from build123d import *

# Parameters (mm, degrees)
SKETCH1_W           = 250
SKETCH1_H           = 150
BOSS_EXTRUDE1_DEPTH = 4
SKETCH2_R           = 20
CUT_EXTRUDE1_DEPTH  = 4
SKETCH3_R           = 2
CUT_EXTRUDE2_DEPTH  = 4
SKETCH4_R           = 14.5
SKETCH4_R_2         = 1.8
CUT_EXTRUDE4_DEPTH  = 4


with BuildPart() as part:
    # Sketch1 → Boss-Extrude1 (new body)
    with BuildSketch(Plane.XY):
        with Locations((12.175324675, -10.633116883)):
            Rectangle(SKETCH1_W, SKETCH1_H)
    extrude(amount=BOSS_EXTRUDE1_DEPTH)

    # Sketch2 → Cut-Extrude1 (cut)
    with BuildSketch(Plane.XY.offset(4)):
        with Locations((12.175324675, -10.633116883)):
            Circle(SKETCH2_R)
    extrude(amount=-CUT_EXTRUDE1_DEPTH, mode=Mode.SUBTRACT)

    # Sketch3 → Cut-Extrude2 (cut)
    with BuildSketch(Plane.XY.offset(4)):
        with Locations((-3.824675325, 5.366883117)):
            Circle(SKETCH3_R)
        with Locations((28.175324675, 5.366883117)):
            Circle(SKETCH3_R)
        with Locations((28.175324675, -26.633116883)):
            Circle(SKETCH3_R)
        with Locations((-3.824675325, -26.633116883)):
            Circle(SKETCH3_R)
    extrude(amount=-CUT_EXTRUDE2_DEPTH, mode=Mode.SUBTRACT)

    # Sketch4 → Cut-Extrude4 (cut)
    with BuildSketch(Plane.XY.offset(4)):
        with Locations((-62.824675325, -55.633116883)):
            Circle(SKETCH4_R)
        with Locations((-74.824675325, -43.633116883)):
            Circle(SKETCH4_R_2)
        with Locations((-50.824675325, -67.633116883)):
            Circle(SKETCH4_R_2)
    extrude(amount=-CUT_EXTRUDE4_DEPTH, mode=Mode.SUBTRACT)


solid = part.part
Can you work these out from the model? Positions are in its coordinate system, mm. Coordinates: 2 decimals unless noted, no trailing zeros. Order: outer loops, then holes, each group sorted by start corner. A loop starts at its lowest first (then second) coordinate and runs counter-clockwise, first axis right, second up. Notation, with made-up numbers: (76, 29) - (131, 29) arc R20 cw to (131, 57) - close; hole circle Ø6 at (33, 83.25). An arc over 180 degrees is marked (long way). Answer as a JSON object with one key per item and string values. Group by question number.
Q1. Imagine slicing it at B-B (z = 2.25). Give the number of separate pieces and of enclosed holes in the cut face, and give its area (3 significant figures).
Q2. We'd pull the mould along X, two halves only. Please class faces 1 (the face through (30.65, -18.29, 2.03)), 2 (the face through (38, -10, 4)): +X half, -X half, draft (parallel to the pull), parting line (faces both ways), or undercut.
Q3. I need wall thicknesses on line 1 (Y direction, x = 21, z = 2.75); line 2 (X direction, y = -67.5, z = 2.6); line 3 (Y direction, x = -57.5, z = 2.1). Which ranges of each line are inside material? Lowest first, please. Write a range as from..to.
Q4. Imagine slicing it at C-C (x = 3). Please give me the cut outline in (y, z).
Q5. Imagine slicing it at A-A (y = -8). Please give me the cut outline in (x, z).
Determined:
{
 "1": {"separate pieces": "1", "enclosed holes": "8", "area": "35,500 mm2"},
 "2": {"face 1": "undercut", "face 2": "draft"},
 "3": {"line 1": "y = -85.63..-28.58, 7.31..64.37", "line 2": "x = -112.82..-71.16, -54.49..-52.62, -49.03..137.18", "line 3": "y = -85.63..-69.12, -42.15..64.37"},
 "4": {"outline": "(-85.63, 0) - (-28.4, 0) - (-28.4, 4) - (-85.63, 4) - close; (7.14, 0) - (64.37, 0) - (64.37, 4) - (7.14, 4) - close"},
 "5": {"outline": "(-112.82, 0) - (-7.65, 0) - (-7.65, 4) - (-112.82, 4) - close; (32, 0) - (137.18, 0) - (137.18, 4) - (32, 4) - close"}
}
